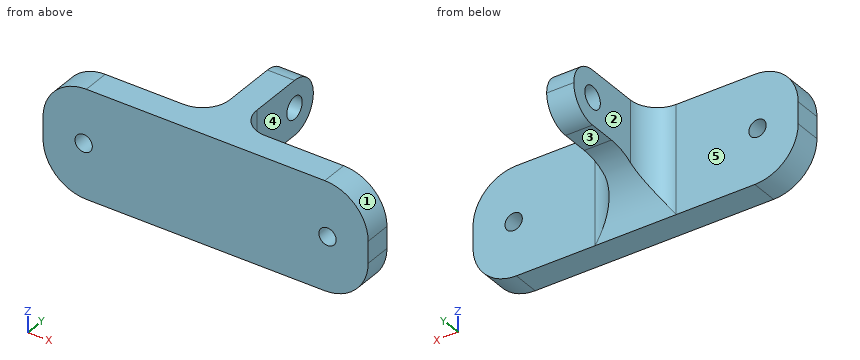
```python
from build123d import *

# Parameters (mm, degrees)
SKETCH_1_W          = 20
SKETCH_1_H          = 15
EXTRUDE_1_DEPTH     = 10
SKETCH_2_W          = 60
SKETCH_2_H          = 20
EXTRUDE_2_DEPTH     = 5
SKETCH_3_R          = 1.6
CUT_EXTRUDE_1_DEPTH = 21
FILLET_1_R          = 8
SKETCH_6_W          = 20
SKETCH_6_H          = 10
CUT_EXTRUDE_3_DEPTH = 10
SKETCH_7_W          = 5
SKETCH_7_H          = 10
EXTRUDE_4_DEPTH     = 20
SKETCH_8_R          = 2.05
CUT_EXTRUDE_4_DEPTH = 20
FILLET_2_R          = 5
FILLET_3_R          = 10
FILLET_4_R          = 5


with BuildPart() as part:
    # 草图1 → 凸台-拉伸1 (new body)
    with BuildSketch(Plane.XY):
        with Locations((10, 7.5)):
            Rectangle(SKETCH_1_W, SKETCH_1_H)
    extrude(amount=EXTRUDE_1_DEPTH)

    # 草图2 → 凸台-拉伸2 (add)
    with BuildSketch(Plane.XZ):
        with Locations((10, 0)):
            Rectangle(SKETCH_2_W, SKETCH_2_H)
    extrude(amount=-EXTRUDE_2_DEPTH)

    # 草图3 → 切除-拉伸1 (cut)
    with BuildSketch(Plane.XZ):
        with Locations(Location((-12.5, 0, 0), (0, 0, 270))):
            Circle(SKETCH_3_R)
        with Locations(Location((32.5, 0, 0), (0, 0, 270))):
            Circle(SKETCH_3_R)
    extrude(amount=-CUT_EXTRUDE_1_DEPTH, mode=Mode.SUBTRACT)

    # 圆角1
    fillet_1_edges = [part.edges().sort_by_distance(p)[0] for p in [
        (-20, 2.5, 10),
        (-20, 2.5, -10),
        (40, 2.5, 10),
        (40, 2.5, -10),
    ]]
    fillet(fillet_1_edges, radius=FILLET_1_R)

    # 草图6 → 切除-拉伸3 (cut)
    with BuildSketch(Plane(origin=(0, 15, 0), x_dir=(1, 0, 0), z_dir=(0, 1, 0))):
        with Locations((10, -5)):
            Rectangle(SKETCH_6_W, SKETCH_6_H)
    extrude(amount=-CUT_EXTRUDE_3_DEPTH, mode=Mode.SUBTRACT)

    # 草图7 → 凸台-拉伸4 (add)
    with BuildSketch(Plane(origin=(0, 5, 0), x_dir=(1, 0, 0), z_dir=(0, 1, 0))):
        with Locations((10, -5)):
            Rectangle(SKETCH_7_W, SKETCH_7_H)
    extrude(amount=EXTRUDE_4_DEPTH)

    # 草图8 → 切除-拉伸4 (cut)
    with BuildSketch(Plane.ZY.offset(-7.5)):
        with Locations((5, 20)):
            Circle(SKETCH_8_R)
    extrude(amount=-CUT_EXTRUDE_4_DEPTH, mode=Mode.SUBTRACT)

    # 圆角2
    fillet_2_edges = [part.edges().sort_by_distance(p)[0] for p in [
        (10, 25, 0),
        (10, 25, 10),
    ]]
    fillet(fillet_2_edges, radius=FILLET_2_R - 0.0001)  # a hair under: the kernel refuses the full size

    # 圆角3
    fillet_3_edges = [part.edges().sort_by_distance(p)[0] for p in [
        (10, 5, 0),
    ]]
    fillet(fillet_3_edges, radius=FILLET_3_R - 0.0001)  # a hair under: the kernel refuses the full size

    # 圆角4
    fillet_4_edges = [part.edges().sort_by_distance(p)[0] for p in [
        (7.5, 5, 5e-05),
        (12.5, 5, 5e-05),
    ]]
    fillet(fillet_4_edges, radius=FILLET_4_R)


solid = part.part
```
Model file for the job. Use its own axes, mm. Face numbers are marked on the shaded views. A direction names the side the tool comes from. Coordinates: 2 decimals unless noted, no trailing zeros. Order: outer loops, then holes, each group sorted by start corner. A loop starts at its lowest first (then second) coordinate and runs counter-clockwise, first axis right, second up. Notation, with made-up numbers: (-0.5, 74) - (29.5, 74) arc R11 cw to (29.5, 91) - close; hole circle Ø5 at (54.25, 74.5). An arc over 180 degrees is marked (long way). Return JSON: item names as keys, results as strings. Group by question number.
1) Saw through at A-A, the plane y = 19.25. Write the cut outline in (x, z).
2) Probe line 1 (X direction, y = 2.3, z = 0); line 2 (X direction, y = 2, z = 1); line 3 (X direction, y = 24, z = 6.25). List the from-to ranges inside material, lowest first. Write a range as from..to.
3) Saw through at C-C, the plane x = 35.5. Write the cut outline in (y, z).
4) Tool access for the marked faces 1, 2, 3, 4 and 5: list every direction of +Z, -Z, +X, -X, +Y, -Y with a clear straight run to the whole face (end or side of a thin tool).
5) Flat gauge pins, fed straight in: P1, Ø10, axis at x = 2.5, z = -3.5, coming from the -Y side; P2, Ø6, axis at y = 7, z = -5, coming from the -X side; P3, Ø12, axis at y = 15.5, z = -4, coming from the -X side; P4, Ø10, axis at x = -8.5, z = -2, coming from the +Y side. Where does each tip first touch, or does it go through?
6) Saw through at B-B, the plane x = -7. Write the cut outline in (y, z), plus the area to 3 significant figures.
Values found:
{
 "1": {"outline": "(7.5, 0) - (12.5, 0) - (12.5, 3.09) - (7.5, 3.09) - close; (7.5, 6.91) - (12.5, 6.91) - (12.5, 10) - (7.5, 10) - close"},
 "2": {"line 1": "x = -20..-14.1, -10.9..30.9, 34.1..40", "line 2": "x = -20..-13.75, -11.25..31.25, 33.75..40", "line 3": "x = 7.5..12.5"},
 "3": {"outline": "(0, -9.19) - (5, -9.19) - (5, 9.19) - (0, 9.19) - close"},
 "4": {"face 1": "+Z, +X, +Y, -Y", "face 2": "+Z, -Z, -X, +Y", "face 3": "-Z, +X, -X, +Y", "face 4": "+Z, -Z, +X, +Y", "face 5": "+Z, -Z, +Y"},
 "5": {"P1": "stops at y = 0", "P2": "stops at x = -19.96", "P3": "stops at x = 7.5", "P4": "stops at y = 5"},
 "6": {"outline": "(0, -10) - (5, -10) - (5, 10) - (0, 10) - close", "area": "100 mm²"}
}
